from build123d import *

# Parameters (mm, degrees)
SKETCH_3_W               = 40
SKETCH_3_H               = 20
EXTRUDE_2_DEPTH          = 39
SKETCH_4_W               = 3
SKETCH_4_H               = 20
EXTRUDE_3_DEPTH          = 5
SKETCH_7_W               = 3
SKETCH_7_H               = 20
EXTRUDE_4_DEPTH          = 5
SKETCH_9_R               = 2
CUT_EXTRUDE_1_DEPTH      = 3
SKETCH_10_R              = 2.009071102
SKETCH_10_R_2            = 2
CUT_EXTRUDE_2_DEPTH      = 3
SKETCH_11_R              = 3
EXTRUDE_6_DEPTH          = 6
SKETCH_16_R              = 6
EXTRUDE_8_DEPTH          = 1.5
SKETCH_17_R              = 7
EXTRUDE_9_DEPTH          = 1
HOLE_WIZARD_3_48_1_D     = 1.9939
HOLE_WIZARD_3_48_1_DEPTH = 3
HOLE_WIZARD_3_48_1_TIP   = 0.599027994


with BuildPart() as part:
    # 草图3 → 凸台-拉伸2 (new body)
    with BuildSketch(Plane.XY):
        with Locations((-53.793598947, 3.253632602)):
            Rectangle(SKETCH_3_W, SKETCH_3_H)
    extrude(amount=EXTRUDE_2_DEPTH)

    # 草图4 → 凸台-拉伸3 (add)
    with BuildSketch(Plane(origin=(-33.793598947, 0, 0), x_dir=(0, 0, -1), z_dir=(1, 0, 0))):
        with Locations((-13.568387962, 3.253632602)):
            Rectangle(SKETCH_4_W, SKETCH_4_H)
    extrude(amount=EXTRUDE_3_DEPTH)

    # 草图7 → 凸台-拉伸4 (add)
    with BuildSketch(Plane.ZY.offset(73.793598947)):
        with Locations((13.473660247, 3.253632602)):
            Rectangle(SKETCH_7_W, SKETCH_7_H)
    extrude(amount=EXTRUDE_4_DEPTH)

    # 草图9 → 切除-拉伸1 (cut)
    with BuildSketch(Plane(origin=(0, 0, 11.973660247), x_dir=(-1, 0, 0), z_dir=(0, 0, -1))):
        with Locations(Location((76.293598947, 9.142056697, 0), (0, 0, 90))):
            Circle(SKETCH_9_R)
        with Locations(Location((76.293598947, -3, 0), (0, 0, 90))):
            Circle(SKETCH_9_R)
    extrude(amount=-CUT_EXTRUDE_1_DEPTH, mode=Mode.SUBTRACT)

    # 草图10 → 切除-拉伸2 (cut)
    with BuildSketch(Plane(origin=(0, 0, 12.068387962), x_dir=(-1, 0, 0), z_dir=(0, 0, -1))):
        with Locations(Location((31.293598947, 9.199024835, 0), (0, 0, 90))):
            Circle(SKETCH_10_R)
        with Locations(Location((31.293598947, -2.746367398, 0), (0, 0, 90))):
            Circle(SKETCH_10_R_2)
    extrude(amount=-CUT_EXTRUDE_2_DEPTH, mode=Mode.SUBTRACT)

    # 草图11 → 凸台-拉伸6 (add)
    with BuildSketch(Plane(origin=(0, 0, 0), x_dir=(-1, 0, 0), z_dir=(0, 0, -1))):
        with Locations(Location((43.293936899, 3.253632602, 0), (0, 0, 180))):
            Circle(SKETCH_11_R)
    extrude(amount=EXTRUDE_6_DEPTH)

    # 草图16 → 凸台-拉伸8 (add)
    with BuildSketch(Plane(origin=(0, 0, 0), x_dir=(-1, 0, 0), z_dir=(0, 0, -1))):
        with Locations(Location((43.293936899, 3.253632602, 0), (0, 0, 180))):
            Circle(SKETCH_16_R)
    extrude(amount=EXTRUDE_8_DEPTH)

    # 草图17 → 凸台-拉伸9 (add)
    with BuildSketch(Plane(origin=(0, 0, 0), x_dir=(-1, 0, 0), z_dir=(0, 0, -1))):
        with Locations(Location((43.293936899, 3.253632602, 0), (0, 0, 180))):
            Circle(SKETCH_17_R)
    extrude(amount=EXTRUDE_9_DEPTH)

    # #3-48 螺纹孔的螺纹孔钻头1
    with Locations(Plane(origin=(0, 0, -6), x_dir=(-1, 0, 0), z_dir=(0, 0, -1))):
        with Locations((43.293936899, 3.253632602)):
            Hole(HOLE_WIZARD_3_48_1_D / 2, depth=HOLE_WIZARD_3_48_1_DEPTH)
            with Locations((0, 0, -(HOLE_WIZARD_3_48_1_DEPTH + HOLE_WIZARD_3_48_1_TIP / 2))):  # 118° drill point
                Cone(0, HOLE_WIZARD_3_48_1_D / 2, HOLE_WIZARD_3_48_1_TIP, mode=Mode.SUBTRACT)


solid = part.part
Geometry: final body of the model. Coordinates: model frame, mm. A direction names the side the tool comes from. Give positions to 0.01 mm unless a question says otherwise; leave off trailing zeros. Loops run counter-clockwise (first coordinate to the right, second up) from the corner with the lowest first, then second, coordinate; pieces in that order, holes last. Notation, with made-up numbers: (31, -3) - (70, -3) arc R15 ccw to (70, 18) - close; hole circle Ø11 at (62.5, 29.25). An arc over 180 degrees is marked (long way). Answer as CSV lines item,"result". Start each with the question number.
1. Section A-A, the plane z = 13.5. Return loops of the section in (x, y).
2. Reachability of faces 4 (the face through (-59, 3, 0)), 5 (the face through (-31, 3, 15.068)), 6 (the face through (-73.794, 3, 6)) from +Z, -Z, +X, -X, +Y, -Y: full face, straight path, thin tool, end or side. Return the list, or none.
3. Section C-C, the plane x = -63.5. Return loops of the section in (y, z).
4. Draft query along X for faces 1 (the face through (-29.31, -3.01, 13.55)), 2 (the face through (-49.29, 2.99, -1.25)), 3 (the face through (-46, 5, -1.5)). Return one class per face: released by +X, released by -X, zero draft, split by the parting line, or undercut.
5. Pin query (flat end, axial travel): P1, Ø4, axis at x = -58, y = 3, coming from the -Z side; P2, Ø1.5, axis at y = 5.5, z = 0, coming from the -X side; P3, Ø1, axis at y = 7.5, z = 6.5, coming from the +X side. Return the tip coordinate at first contact, or that it passes through.
6. Ray query, L1, parallel to X at y = 7, z = 23; L2, parallel to Z at x = -57, y = 0; L3, parallel to Z at x = -76.5, y = 6.75. Return the intervals inside material, ascending.
7. Section D-D, the plane z = 33.5. Return loops of the section in (x, y), plus the area to 3 significant figures.
8. Section B-B, the plane y = 5.5. Return loops of the section in (x, z).
Answers:
1,outline,"(-78.79, -6.75) - (-28.79, -6.75) - (-28.79, 13.25) - (-78.79, 13.25) - close; hole circle Ø4 at (-76.29, -3); hole circle Ø4 at (-76.29, 9.14); hole circle Ø4.02 at (-31.29, 9.2); hole circle Ø4 at (-31.29, -2.75)"
2,face 4,"-Z"
2,face 5,"+Z, +X, +Y, -Y"
2,face 6,"-Z, -X, +Y, -Y"
3,outline,"(-6.75, 0) - (13.25, 0) - (13.25, 39) - (-6.75, 39) - close"
4,face 1,"undercut"
4,face 2,"split by the parting line"
4,face 3,"zero draft"
5,P1,"stops at z = 0"
5,P2,"stops at x = -73.79"
5,P3,"stops at x = -33.79"
6,L1,"x = -73.79 to -33.79"
6,L2,"z = 0 to 39"
6,L3,"z = 11.97 to 14.97"
7,outline,"(-73.79, -6.75) - (-33.79, -6.75) - (-33.79, 13.25) - (-73.79, 13.25) - close"
7,area,"800 mm2"
8,outline,"(-78.79, 11.97) - (-73.79, 11.97) - (-73.79, 0) - (-49.92, 0) - (-49.92, -1) - (-48.86, -1) - (-48.86, -1.5) - (-45.28, -1.5) - (-45.28, -6) - (-41.31, -6) - (-41.31, -1.5) - (-37.73, -1.5) - (-37.73, -1) - (-36.66, -1) - (-36.66, 0) - (-33.79, 0) - (-33.79, 12.07) - (-28.79, 12.07) - (-28.79, 15.07) - (-33.79, 15.07) - (-33.79, 39) - (-73.79, 39) - (-73.79, 14.97) - (-78.79, 14.97) - close"
